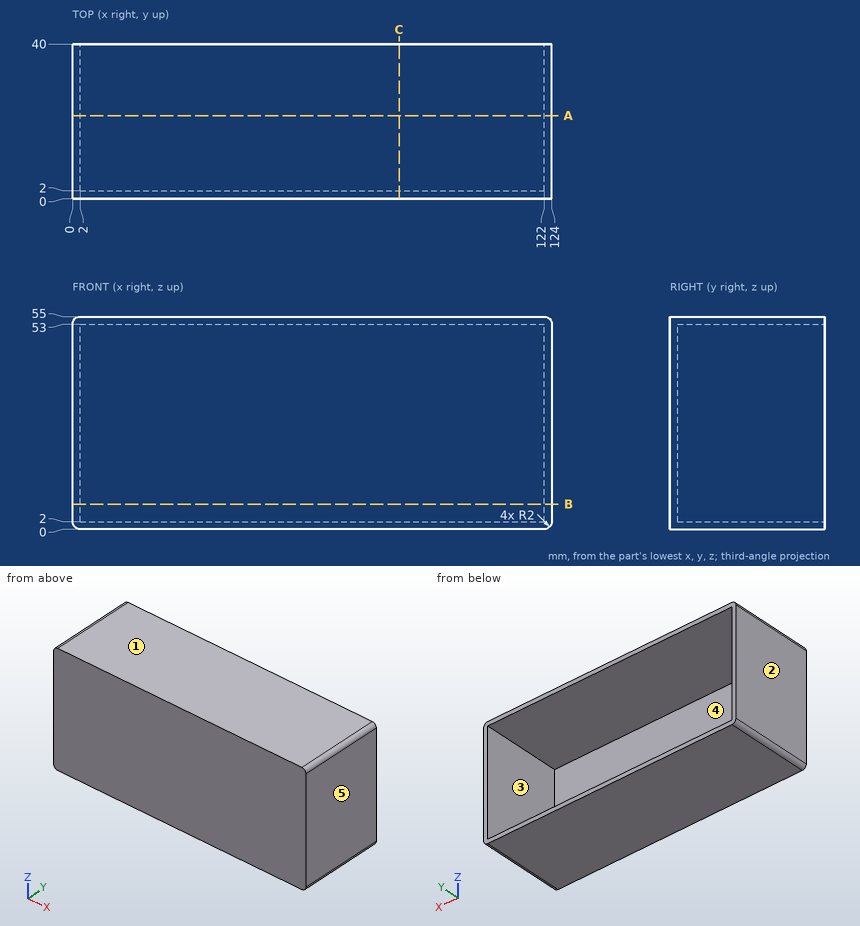
The figure shows three views and two pictorial views of one solid part (mm, origin at its lowest corner). Answer the questions. A direction names the side the tool comes from. Round coordinates to 2 decimals unless told otherwise and drop trailing zeros. Write each loop counter-clockwise with the first axis right and the second up, starting at its lowest first coordinate (ties: lowest second). Pieces come first, ordered by that corner, then holes. Notation, with made-up numbers: (2.25, 37) - (52.25, 37) arc R33 cw to (52.25, 70) - close; hole circle Ø8 at (-14.5, 26). An arc over 180 degrees is marked (long way). One line per question, with ' | ' between items. Start each with the question number.
1. Section C-C (x = 84.5) is taken. Determine the outline of the cut face in (y, z).
2. This flat-tipped pin is pushed along its axis until it touches: pin 1 (5 mm diameter, centred on x = 19.5, z = 11, fed in from +Y). Where does it stop, or does it pass through?
3. Section B-B (z = 6.5) is taken. Determine the outline of the cut face in (x, y).
4. For a pull along X with two mould halves and no side action, classify the marked faces 1, 2 and 3 as +X half, -X half, draft (parallel to the pull), parting line (faces both ways), or undercut.
5. Section A-A (y = 21.5) is taken. Determine the outline of the cut face in (x, z).
6. For the marked faces 4 and 5, determine the directions among +Z, -Z, +X, -X, +Y, -Y from which every point of the face is accessible in a straight line to the end or side of a thin tool.
7. Find the intervals of material crossed by probe 1 along Z at (x, y) = (63, 11); probe 2 along X at (y, z) = (22, 3.5); probe 3 along Y at (x, z) = (31.5, 45.5), in increasing order. Write a range as [from, to].
Filled in:
1) outline: (0, 0) - (40, 0) - (40, 2) - (2, 2) - (2, 53) - (40, 53) - (40, 55) - (0, 55) - close
2) pin 1: y = 2
3) outline: (0, 0) - (124, 0) - (124, 40) - (122, 40) - (122, 2) - (2, 2) - (2, 40) - (0, 40) - close
4) face 1: draft | face 2: -X half | face 3: undercut
5) outline: (0, 2) arc R2 ccw to (2, 0) - (122, 0) arc R2 ccw to (124, 2) - (124, 53) arc R2 ccw to (122, 55) - (2, 55) arc R2 ccw to (0, 53) - close; hole (2, 2) - (122, 2) - (122, 53) - (2, 53) - close
6) face 4: +Y | face 5: +Z, -Z, +X, +Y, -Y
7) probe 1: [0, 2], [53, 55] | probe 2: [0, 2], [122, 124] | probe 3: [0, 2]
